```python
from build123d import *

# Parameters (mm, degrees)
SKETCH2_R           = 25
BOSS_EXTRUDE1_DEPTH = 10
SKETCH4_R           = 11.25
SKETCH4_W           = 12
SKETCH4_H           = 6
CUT_EXTRUDE1_DEPTH  = 87.602540378
FILLET1_R           = 0.2
CHAMFER1_SIZE       = 1
CHAMFER2_SIZE       = 1


with BuildPart() as part:
    # Sketch1 → Revolve12 (revolve)
    with BuildSketch(Plane.XY, mode=Mode.PRIVATE) as revolve12_sk:
        Polygon((3, 50), (-3, 50), (-6.639702343, 40), (-10.360297657, 40), (-14, 50), (-20, 50), (-20, 0), (20, 0), (20, 50), (14, 50), (10.360297657, 40), (6.639702343, 40), align=None)
    revolve(revolve12_sk.sketch.rotate(Axis((-20, 0, 0), (1, 0, 0)), 180), axis=Axis((-20, 0, 0), (1, 0, 0)))

    # Sketch2 → Boss-Extrude1 (add)
    with BuildSketch(Plane.ZY.offset(20)):
        with Locations(Location((0, 0, 0), (0, 0, 90))):
            Circle(SKETCH2_R)
    extrude(amount=BOSS_EXTRUDE1_DEPTH)

    # Sketch4 → Cut-Extrude1 (cut, through all)
    with BuildSketch(Plane.ZY.offset(30)):
        Circle(SKETCH4_R)
        with Locations((0, 11.25)):
            Rectangle(SKETCH4_W, SKETCH4_H)
    extrude(amount=-CUT_EXTRUDE1_DEPTH, mode=Mode.SUBTRACT)

    # Fillet1
    fillet1_edges = [part.edges().sort_by_distance(p)[0] for p in [
        (-20, -25, 0),
    ]]
    fillet(fillet1_edges, radius=FILLET1_R)

    # Chamfer1
    chamfer1_edges = [part.edges().sort_by_distance(p)[0] for p in [
        (20, -11.25, 0),
    ]]
    chamfer(chamfer1_edges, length=CHAMFER1_SIZE)

    # Chamfer2
    chamfer2_edges = [part.edges().sort_by_distance(p)[0] for p in [
        (-30, -11.25, 0),
    ]]
    chamfer(chamfer2_edges, length=CHAMFER2_SIZE)


solid = part.part
```
Work out the finished part from the listing and answer in its coordinate system (mm). A direction names the side the tool comes from. Round coordinates to 2 decimals unless told otherwise and drop trailing zeros. Loops run counter-clockwise (first coordinate to the right, second up) from the corner with the lowest first, then second, coordinate; pieces in that order, holes last. Notation, with made-up numbers: M -13,25 L 36,25 A17 cw 36,34 Z; hole C 37.25,35.5 d2. An arc over 180 degrees is marked long. One line per question, with ' | ' between items.
Q1. Find section D-D, the plane y = -43. State how many separate pieces and enclosed holes the cut face has, then the cut area to 3 significant figures.
Conclusion:
separate pieces: 3 | enclosed holes: 0 | area: 1,260 mm2
Q2. A tool of negligible diameter and unlimited length cuts with its end or side. For faces 4 (the flat face through (-5, 14.25, 0)), 5 (the flat face through (20, 10, 10)), 6 (the flat face through (-20, 12, -23)), 7 (the cylindrical face through (8.47, 39.96, -1.76)), from which of +Z, -Z, +X, -X, +Y, -Y can it reach the whole face along a straight path? Write none if from no direction.
Conclusion:
face 4: +X, -X | face 5: +Z, -Z, +X, +Y, -Y | face 6: -X | face 7: none
Q3. Find section C-C, the plane x = -16.5. Give the vertices of the cut face in (y, z).
Conclusion:
outline: C 0,0 d100; hole M 9.52,-6 L 14.25,-6 L 14.25,6 L 9.52,6 A11.25 ccw long Z
Q4. Consider line 1 along Z through (x, y) = (-9, 0); line 2 along X through (y, z) = (18.5, -41); line 3 along X through (y, z) = (-12, -40). Determine where each line is inside the solid, lowest interval first. Write a range as from..to.
Conclusion:
line 1: z = -40..-11.25, 11.25..40 | line 2: x = -20..-12.17, -4.83..4.83, 12.17..20 | line 3: x = -20..-11, -6..6, 11..20
Q5. The mould has two halves that part along Z. Classify faces 1 (the conical face through (19.174, -11.416, -0.42)), 2 (the cylindrical face through (16.96, -47.69, -15.02)), 3 (the flat face through (-30, -6, 11)): +Z half, -Z half, draft (parallel to the pull), parting line (faces both ways), or undercut.
Conclusion:
face 1: undercut | face 2: parting line | face 3: draft
Q6. Each of these flat-tipped pins is pushed along its axis until it touches: pin 1 Ø4 at (y, z) = (-18, 33) entering from -X; pin 2 Ø5 at (x, z) = (-5, -2.5) entering from +Y; pin 3 Ø2.5 at (x, y) = (-3.5, 12) entering from -Z. Where does it stop, or does it pass through?
Conclusion:
pin 1: stops at x = -20 | pin 2: stops at y = 49.99 | pin 3: stops at z = -48.81
